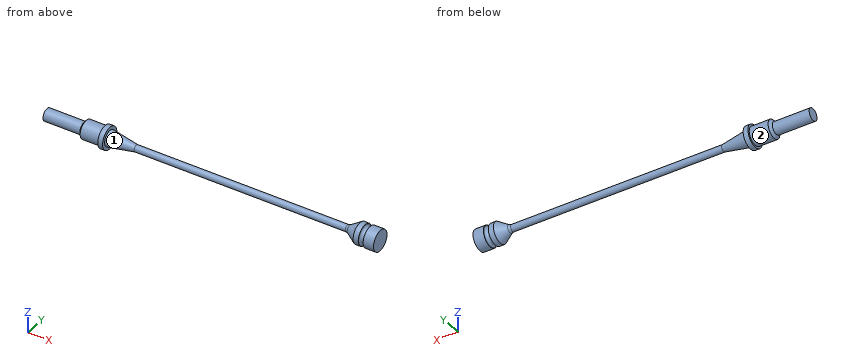
```python
from build123d import *


with BuildPart() as part:
    # Sketch2 → Revolve2 (revolve)
    with BuildSketch(Plane.XY, mode=Mode.PRIVATE) as revolve2_sk:
        with BuildLine():
            Line((190.5, 0), (190.5, 5.98805))
            Line((190.5, 5.98805), (184.5564, 5.98805))
            Line((184.5564, 5.98805), (184.5564, 5.588))
            ThreePointArc((184.5564, 5.588), (183.1594, 4.191), (181.7624, 5.588))
            Line((181.7624, 5.588), (181.7624, 5.98805))
            Line((181.7624, 5.98805), (178.8287, 5.98805))
            Line((178.8287, 5.98805), (173.106298001, 2.308545514))
            ThreePointArc((173.106298001, 2.308545514), (172.448450778, 2.007973698), (171.732557766, 1.905))
            Line((171.732557766, 1.905), (51.082557766, 1.905))
            Line((51.082557766, 1.905), (35.8775, 4.51485))
            Line((35.8775, 4.51485), (35.8775, 6.35))
            Line((35.8775, 6.35), (33.1343, 6.35))
            Line((33.1343, 6.35), (33.1343, 5.22605))
            Line((33.1343, 5.22605), (22.352, 5.22605))
            Line((22.352, 5.22605), (21.082, 3.48615))
            Line((21.082, 3.48615), (0, 3.48615))
            Line((0, 3.48615), (0, 0))
            Line((0, 0), (190.5, 0))
        make_face()
    revolve(revolve2_sk.sketch.rotate(Axis((0, 0, 0), (1, 0, 0)), 90), axis=Axis((0, 0, 0), (1, 0, 0)))


solid = part.part
```
Check sheet for the modelled part. Datum: model origin and axes. Units: mm. Face numbers are marked on the shaded views. Give positions to 0.01 mm unless a question says otherwise; leave off trailing zeros. Order: outer loops, then holes, each group sorted by start corner. A loop starts at its lowest first (then second) coordinate and runs counter-clockwise, first axis right, second up. Notation, with made-up numbers: M -19,85.25 L 14,85.25 A9 ccw 14,91.25 Z; hole C -1.5,-3.75 d7. An arc over 180 degrees is marked long. Answer in a Markdown table with one row per item.
1) Gauge pin test, flat ends, axial feed: P1, Ø4, axis at x = 45, z = -3, coming from the -Y side; P2, Ø1.5, axis at x = 91.5, z = 0.5, coming from the -Y side (3 decimals); P3, Ø4, axis at x = 74, y = -3, coming from the -Z side. Record the tip position at first contact, or that the pin passes through.
Filled sheet:
| item | result |
|---|---|
| P1 | stops at y = -2.86 |
| P2 | stops at y = -1.905 |
| P3 | stops at z = -1.62 |
2) Release check for a two-part mould opening along X. For the marked faces 1 and 2 record: +X half, -X half, draft (parallel to the pull), parting line (faces both ways), or undercut.
Filled sheet:
| item | result |
|---|---|
| face 1 | undercut |
| face 2 | draft |
3) Cross-section at C-C, the plane x = 104. Enter the section's corners in (y, z) (3 decimals).
Filled sheet:
| item | result |
|---|---|
| outline | C 0,0 d3.81 |
4) Thickness scan on L1, parallel to X at y = 0.5, z = 5; L2, parallel to X at y = 1.5, z = -5.25; L3, parallel to Y at x = 84, z = -0.25. Record the ranges inside material, lowest first. Write a range as [from, to].
Filled sheet:
| item | result |
|---|---|
| L1 | x = [22.21, 35.88], [177.33, 181.88], [184.44, 190.5] |
| L2 | x = [33.13, 35.88], [178.01, 181.77], [184.55, 190.5] |
| L3 | y = [-1.89, 1.89] |
